Design review of the part shown in the three views and the two pictorial views. Dimensions are in mm from the part's minimum x, y and z. A direction names the side the tool comes from. Round coordinates to 2 decimals unless told otherwise and drop trailing zeros. Order: outer loops, then holes, each group sorted by start corner. A loop starts at its lowest first (then second) coordinate and runs counter-clockwise, first axis right, second up. Notation, with made-up numbers: M 10,-1 L 55,-1 A27 ccw 55,33 Z; hole C -15.5,42.25 d8. An arc over 180 degrees is marked long. Use a Markdown table: item, result. Add a question column.
(1) For pin 1 (12 mm diameter, centred on x = 123.5, y = 18, fed in from +Z); pin 2 (15.5 mm diameter, centred on x = 10, z = 110, fed in from -Y); pin 3 (6 mm diameter, centred on x = 251.5, y = 5.5, fed in from +Z); pin 4 (7 mm diameter, centred on x = 50.68, z = 34.72, fed in from -Y), all flat-tipped, find the tip position at first contact; note any pin that passes through.
(2) The part is to be moulded in two halves that separate along X. For the marked faces 1, 2 and 3, say which applies: released by +X, released by -X, zero draft, split by the parting line, or undercut.
(3) To check wall thickness, follow probe 1 along Z at (x, y) = (100, 13.5); probe 2 along X at (y, z) = (6.75, 87); probe 3 along X at (y, z) = (6.25, 112.5). State the ranges of each line that lie inside material, in increasing order. Write a range as from..to.
(4) Machinability: for the marked faces 4, 5 and 6, which of the approach directions +Z, -Z, +X, -X, +Y, -Y give a long, thin tool a straight path to every point of the face, cutting with its end or side? Answer none if there is none.
(5) Take a section at D-D (y = 4). Write out the cut boundary in (x, z).
(6) Take a section at C-C (z = 46). Write out the cut boundary in (x, y).
(7) Take a section at B-B (x = 250). Write out the cut boundary in (y, z).
(8) Take a section at A-A (z = 110). Write out the cut boundary in (x, y).
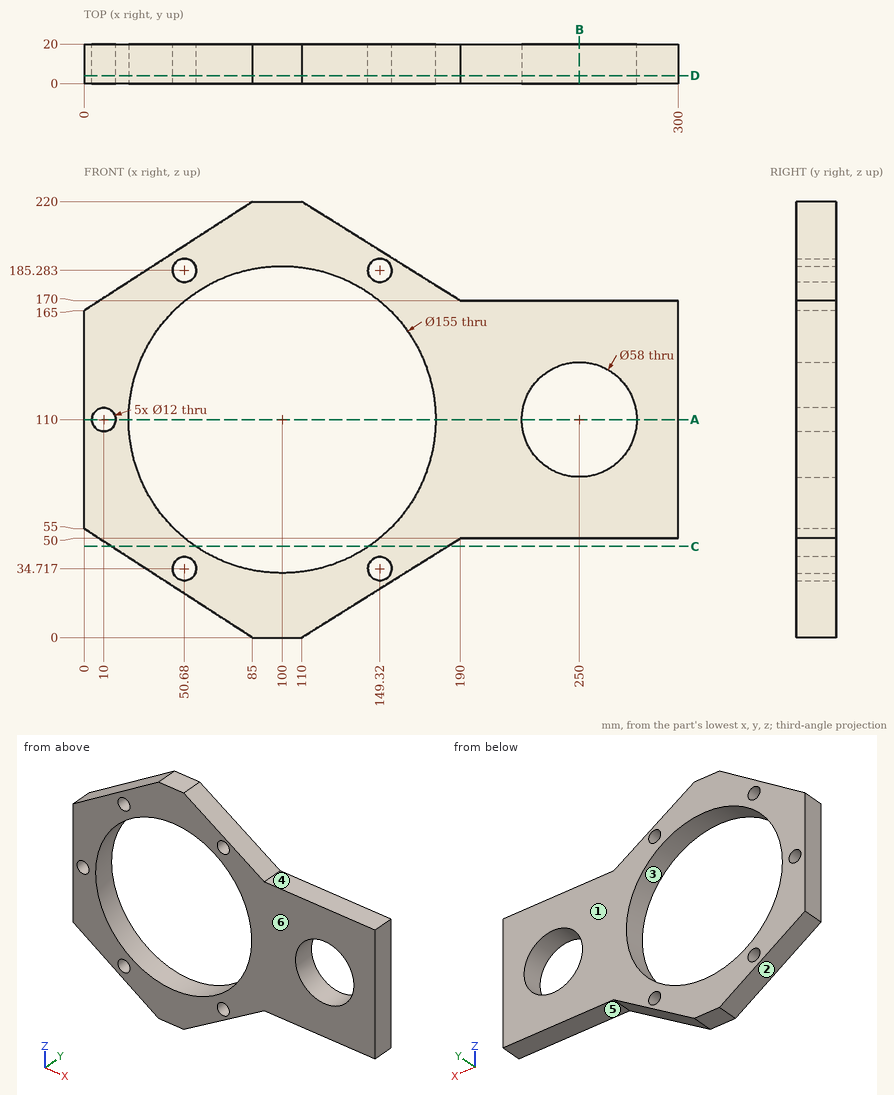
Verdict:
| question | item | result |
|---|---|---|
| 1 | pin 1 | stops at z = 215.31 |
| 1 | pin 2 | stops at y = 0 |
| 1 | pin 3 | stops at z = 170 |
| 1 | pin 4 | passes through |
| 2 | face 1 | zero draft |
| 2 | face 2 | released by -X |
| 2 | face 3 | undercut |
| 3 | probe 1 | z = 0..32.5, 187.5..220 |
| 3 | probe 2 | x = 0..25.99, 174.01..232.34, 267.66..300 |
| 3 | probe 3 | x = 0..4.55, 15.45..22.54, 177.46..221.11, 278.89..300 |
| 4 | face 4 | +Z, +X, +Y, -Y |
| 4 | face 5 | -Z, +X, +Y, -Y |
| 4 | face 6 | +Z, -Z, +X, -X, -Y |
| 5 | outline | M 0,55 L 85,0 L 110,0 L 190,50 L 300,50 L 300,170 L 190,170 L 110,220 L 85,220 L 0,165 Z; hole C 10,110 d12; hole C 100,110 d155; hole C 50.68,34.72 d12; hole C 50.68,185.28 d12; hole C 149.32,34.72 d12; hole C 149.32,185.28 d12; hole C 250,110 d58 |
| 6 | outline | M 13.91,0 L 56.29,0 L 56.29,20 L 13.91,20 Z; M 143.71,0 L 183.6,0 L 183.6,20 L 143.71,20 Z |
| 7 | outline | M 0,50 L 20,50 L 20,81 L 0,81 Z; M 0,139 L 20,139 L 20,170 L 0,170 Z |
| 8 | outline | M 0,0 L 4,0 L 4,20 L 0,20 Z; M 16,0 L 22.5,0 L 22.5,20 L 16,20 Z; M 177.5,0 L 221,0 L 221,20 L 177.5,20 Z; M 279,0 L 300,0 L 300,20 L 279,20 Z |
